Design review of the part shown in the three views and the two pictorial views. Dimensions are in mm from the part's minimum x, y and z. A direction names the side the tool comes from. Give positions to 0.01 mm unless a question says otherwise; leave off trailing zeros. Loops run counter-clockwise (first coordinate to the right, second up) from the corner with the lowest first, then second, coordinate; pieces in that order, holes last. Notation, with made-up numbers: (-30, 76.25) - (-3, 76.25) arc R21 cw to (-3, 114.25) - close; hole circle Ø7 at (-5.5, 74.5). An arc over 180 degrees is marked (long way). Answer as a JSON object with one key per item and string values.
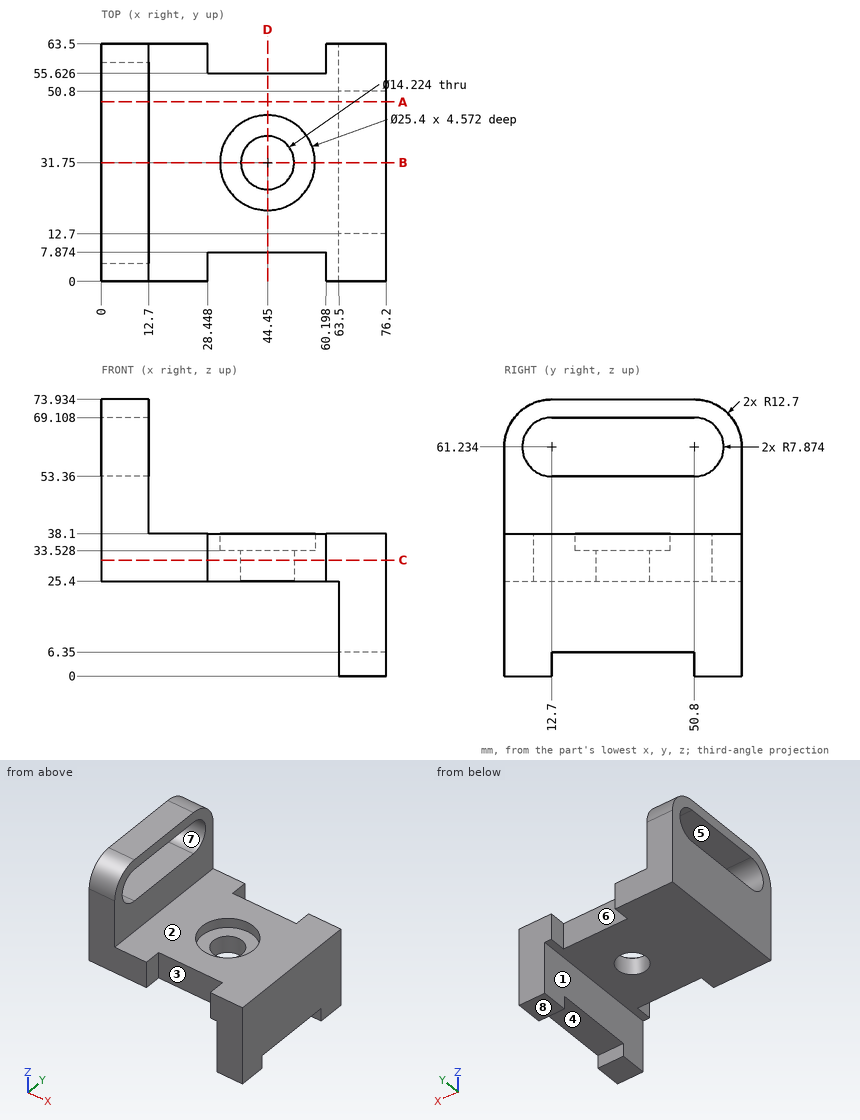
Q1. Clearance check with flat-ended pins moving along their axes: pin 1 Ø7 at (x, z) = (71, 4) entering from -Y; pin 2 Ø4 at (x, y) = (6.5, 36.5) entering from -Z; pin 3 Ø14 at (x, y) = (68, 37.5) entering from -Z; pin 4 Ø20.5 at (x, y) = (44, 30) entering from +Z. State where each tip first meets the part, or that it passes through.
Results:
{"pin 1": "stops at y = 0", "pin 2": "stops at z = 25.4", "pin 3": "stops at z = 6.35", "pin 4": "stops at z = 33.53"}
Q2. For the marked faces 1, 2, 3, 4 and 5, list the 3-axis set-ups (+Z, -Z, +X, -X, +Y, -Y) from which the entire face can be reached by the end or side of a thin tool; tool diameter is ignored.
Results:
{"face 1": "-Z, -X, +Y, -Y", "face 2": "+Z, +X, +Y, -Y", "face 3": "+Z, -Z, -Y", "face 4": "-Z, +X, -X", "face 5": "+X, -X"}
Q3. Consider section B-B, the plane y = 31.75. State the section outline as (x, z) points.
Results:
{"outline": "(0, 25.4) - (37.34, 25.4) - (37.34, 33.53) - (31.75, 33.53) - (31.75, 38.1) - (12.7, 38.1) - (12.7, 53.36) - (0, 53.36) - close; (0, 69.11) - (12.7, 69.11) - (12.7, 73.93) - (0, 73.93) - close; (51.56, 25.4) - (63.5, 25.4) - (63.5, 6.35) - (76.2, 6.35) - (76.2, 38.1) - (57.15, 38.1) - (57.15, 33.53) - (51.56, 33.53) - close"}
Q4. Consider section A-A, the plane y = 48. State the section outline as (x, z) points.
Results:
{"outline": "(0, 25.4) - (63.5, 25.4) - (63.5, 6.35) - (76.2, 6.35) - (76.2, 38.1) - (12.7, 38.1) - (12.7, 53.36) - (0, 53.36) - close; (0, 69.11) - (12.7, 69.11) - (12.7, 73.93) - (0, 73.93) - close"}
Q5. To check wall thickness, follow probe 1 along Y at (x, z) = (44, 28); probe 2 along Y at (x, z) = (44.45, 29); probe 3 along X at (y, z) = (53, 9). State the ranges of each line that lie inside material, in increasing order. Write a range as [from, to].
Results:
{"probe 1": "y = [7.87, 24.65], [38.85, 55.63]", "probe 2": "y = [7.87, 24.64], [38.86, 55.63]", "probe 3": "x = [63.5, 76.2]"}
Q6. Consider section D-D, the plane x = 44.45. State the section outline as (y, z) points, plus the area to 3 significant figures.
Results:
{"outline": "(7.87, 25.4) - (24.64, 25.4) - (24.64, 33.53) - (19.05, 33.53) - (19.05, 38.1) - (7.87, 38.1) - close; (38.86, 25.4) - (55.63, 25.4) - (55.63, 38.1) - (44.45, 38.1) - (44.45, 33.53) - (38.86, 33.53) - close", "area": "375 mm^2"}
Q7. Consider section C-C, the plane z = 31. State the section outline as (x, y) points.
Results:
{"outline": "(0, 0) - (28.45, 0) - (28.45, 7.87) - (60.2, 7.87) - (60.2, 0) - (76.2, 0) - (76.2, 63.5) - (60.2, 63.5) - (60.2, 55.63) - (28.45, 55.63) - (28.45, 63.5) - (0, 63.5) - close; hole circle Ø14.22 at (44.45, 31.75)"}
Q8. The part is to be moulded in two halves that separate along Y. For the marked faces 6, 7 and 8, say which applies: +Y half, -Y half, draft (parallel to the pull), parting line (faces both ways), or undercut.
Results:
{"face 6": "+Y half", "face 7": "undercut", "face 8": "draft"}
